CAD build for the part. Positions are in the model's coordinates, mm. A direction names the side the tool comes from. Give positions to 0.01 mm unless a question says otherwise; leave off trailing zeros. Order: outer loops, then holes, each group sorted by start corner. A loop starts at its lowest first (then second) coordinate and runs counter-clockwise, first axis right, second up. Notation, with made-up numbers: M 36,-17.5 L 67,-17.5 A25 ccw 67,-4.5 Z; hole C -19,35 d9. An arc over 180 degrees is marked long. Put each result on its own line as item: value. Start each with the question number.
1) Drill centre lines: line 1 (X direction, y = -157.7, z = 5.25); line 2 (X direction, y = -105, z = 0.75); line 3 (Y direction, x = 27, z = 8.25). Where is each one in solid material? Low to high. Write a range as [from, to].
2) Cut at A-A (x = 40). Write the cut outline in (y, z).
3) Cut at D-D (y = -104). Write the cut outline in (x, z).
4) Pin check, flat tips, straight feed: pin 1 (5 mm diameter, centred on x = -56.505, y = -54.325, fed in from -Z); pin 2 (1 mm diameter, centred on y = -138, z = 1, fed in from -X); pin 3 (1.5 mm diameter, centred on y = -124, z = 4, fed in from +X); pin 4 (5 mm diameter, centred on x = -52, z = 5, fed in from -Y). Stop position of each tip, or through.
5) Cut at C-C (z = 4.5). Give the number of separate pieces and of enclosed holes in the cut face, and give its area (3 significant figures).
6) Two-plate mould, pull along Y, no slides. Class faces 1 (the face through (-1, -23, 9.53)), 2 (the face through (62, -62.5, 5)), 3 (the face through (-38.85, -159.92, 4.83)): released by +Y, released by -Y, zero draft, split by the parting line, or undercut.
7) Cut at B-B (y = -157.7). Write the cut outline in (x, z), and give its area (3 significant figures).
8) Tool access for faces 4 (the face through (45, -115, 5)), 5 (the face through (-1, -23, 0)), 6 (the face through (-62, -62.5, 5)): list every direction of +Z, -Z, +X, -X, +Y, -Y with a clear straight run to the whole face (end or side of a thin tool).
```python
from build123d import *

# Parameters (mm, degrees)
RESSALTO_EXTRUS_O1_DEPTH = 9.53
CORTE_EXTRUS_O1_REACH    = 179.792
ESBO_O2_R                = 2.5
CORTE_EXTRUS_O2_REACH    = 179.792
ESBO_O3_R                = 1.5
CROQUIS1_W               = 1
CROQUIS1_H               = 125
SALIENTE_EXTRUIR1_DEPTH  = 9.53
REDONDEO1_R              = 6


with BuildPart() as part:
    # Esboço1 → Ressalto-extrusão1 (new body)
    with BuildSketch(Plane.XY):
        Polygon((-71.505, 62.5), (71.505, 62.5), (71.505, -62.5), (45, -62.5), (45, -162.5), (-45, -162.5), (-45, -62.5), (-71.505, -62.5), align=None)
    extrude(amount=RESSALTO_EXTRUS_O1_DEPTH)

    # Esboço2 → Corte-extrusão1 (cut, up to next)
    with BuildSketch(Plane.XY.offset(9.53), mode=Mode.PRIVATE) as corte_extrus_o1_sk1:
        with Locations((-40, -157.7)):
            Circle(ESBO_O2_R)
    corte_extrus_o1_tool1 = extrude(corte_extrus_o1_sk1.sketch, amount=-CORTE_EXTRUS_O1_REACH, mode=Mode.PRIVATE) & part.part
    # Esboço2 → Corte-extrusão1 (cut, up to next)
    with BuildSketch(Plane.XY.offset(9.53), mode=Mode.PRIVATE) as corte_extrus_o1_sk2:
        with Locations((-25, -157.7)):
            Circle(ESBO_O2_R)
    corte_extrus_o1_tool2 = extrude(corte_extrus_o1_sk2.sketch, amount=-CORTE_EXTRUS_O1_REACH, mode=Mode.PRIVATE) & part.part
    # Esboço2 → Corte-extrusão1 (cut, up to next)
    with BuildSketch(Plane.XY.offset(9.53), mode=Mode.PRIVATE) as corte_extrus_o1_sk3:
        with Locations((25, -157.7)):
            Circle(ESBO_O2_R)
    corte_extrus_o1_tool3 = extrude(corte_extrus_o1_sk3.sketch, amount=-CORTE_EXTRUS_O1_REACH, mode=Mode.PRIVATE) & part.part
    # Esboço2 → Corte-extrusão1 (cut, up to next)
    with BuildSketch(Plane.XY.offset(9.53), mode=Mode.PRIVATE) as corte_extrus_o1_sk4:
        with Locations((40, -157.7)):
            Circle(ESBO_O2_R)
    corte_extrus_o1_tool4 = extrude(corte_extrus_o1_sk4.sketch, amount=-CORTE_EXTRUS_O1_REACH, mode=Mode.PRIVATE) & part.part
    # Esboço2 → Corte-extrusão1 (cut, up to next)
    with BuildSketch(Plane.XY.offset(9.53), mode=Mode.PRIVATE) as corte_extrus_o1_sk5:
        with Locations((40, -98.2)):
            Circle(ESBO_O2_R)
    corte_extrus_o1_tool5 = extrude(corte_extrus_o1_sk5.sketch, amount=-CORTE_EXTRUS_O1_REACH, mode=Mode.PRIVATE) & part.part
    # Esboço2 → Corte-extrusão1 (cut, up to next)
    with BuildSketch(Plane.XY.offset(9.53), mode=Mode.PRIVATE) as corte_extrus_o1_sk6:
        with Locations((25, -98.2)):
            Circle(ESBO_O2_R)
    corte_extrus_o1_tool6 = extrude(corte_extrus_o1_sk6.sketch, amount=-CORTE_EXTRUS_O1_REACH, mode=Mode.PRIVATE) & part.part
    # Esboço2 → Corte-extrusão1 (cut, up to next)
    with BuildSketch(Plane.XY.offset(9.53), mode=Mode.PRIVATE) as corte_extrus_o1_sk7:
        with Locations((-25, -98.2)):
            Circle(ESBO_O2_R)
    corte_extrus_o1_tool7 = extrude(corte_extrus_o1_sk7.sketch, amount=-CORTE_EXTRUS_O1_REACH, mode=Mode.PRIVATE) & part.part
    # Esboço2 → Corte-extrusão1 (cut, up to next)
    with BuildSketch(Plane.XY.offset(9.53), mode=Mode.PRIVATE) as corte_extrus_o1_sk8:
        with Locations((-40, -98.2)):
            Circle(ESBO_O2_R)
    corte_extrus_o1_tool8 = extrude(corte_extrus_o1_sk8.sketch, amount=-CORTE_EXTRUS_O1_REACH, mode=Mode.PRIVATE) & part.part
    add(corte_extrus_o1_tool1.solids().sort_by_distance((-40, -157.7, 9.53))[0], mode=Mode.SUBTRACT)
    add(corte_extrus_o1_tool2.solids().sort_by_distance((-25, -157.7, 9.53))[0], mode=Mode.SUBTRACT)
    add(corte_extrus_o1_tool3.solids().sort_by_distance((25, -157.7, 9.53))[0], mode=Mode.SUBTRACT)
    add(corte_extrus_o1_tool4.solids().sort_by_distance((40, -157.7, 9.53))[0], mode=Mode.SUBTRACT)
    add(corte_extrus_o1_tool5.solids().sort_by_distance((40, -98.2, 9.53))[0], mode=Mode.SUBTRACT)
    add(corte_extrus_o1_tool6.solids().sort_by_distance((25, -98.2, 9.53))[0], mode=Mode.SUBTRACT)
    add(corte_extrus_o1_tool7.solids().sort_by_distance((-25, -98.2, 9.53))[0], mode=Mode.SUBTRACT)
    add(corte_extrus_o1_tool8.solids().sort_by_distance((-40, -98.2, 9.53))[0], mode=Mode.SUBTRACT)

    # Esboço3 → Corte-extrusão2 (cut, up to next)
    with BuildSketch(Plane(origin=(0, 0, 0), x_dir=(-1, 0, 0), z_dir=(0, 0, -1)), mode=Mode.PRIVATE) as corte_extrus_o2_sk1:
        with Locations((56.505, -54.325)):
            Circle(ESBO_O3_R)
    corte_extrus_o2_tool1 = extrude(corte_extrus_o2_sk1.sketch, amount=-CORTE_EXTRUS_O2_REACH, mode=Mode.PRIVATE) & part.part
    # Esboço3 → Corte-extrusão2 (cut, up to next)
    with BuildSketch(Plane(origin=(0, 0, 0), x_dir=(-1, 0, 0), z_dir=(0, 0, -1)), mode=Mode.PRIVATE) as corte_extrus_o2_sk2:
        with Locations((26.505, -54.325)):
            Circle(ESBO_O3_R)
    corte_extrus_o2_tool2 = extrude(corte_extrus_o2_sk2.sketch, amount=-CORTE_EXTRUS_O2_REACH, mode=Mode.PRIVATE) & part.part
    # Esboço3 → Corte-extrusão2 (cut, up to next)
    with BuildSketch(Plane(origin=(0, 0, 0), x_dir=(-1, 0, 0), z_dir=(0, 0, -1)), mode=Mode.PRIVATE) as corte_extrus_o2_sk3:
        with Locations((-26.505, -54.325)):
            Circle(ESBO_O3_R)
    corte_extrus_o2_tool3 = extrude(corte_extrus_o2_sk3.sketch, amount=-CORTE_EXTRUS_O2_REACH, mode=Mode.PRIVATE) & part.part
    # Esboço3 → Corte-extrusão2 (cut, up to next)
    with BuildSketch(Plane(origin=(0, 0, 0), x_dir=(-1, 0, 0), z_dir=(0, 0, -1)), mode=Mode.PRIVATE) as corte_extrus_o2_sk4:
        with Locations((-56.505, -54.325)):
            Circle(ESBO_O3_R)
    corte_extrus_o2_tool4 = extrude(corte_extrus_o2_sk4.sketch, amount=-CORTE_EXTRUS_O2_REACH, mode=Mode.PRIVATE) & part.part
    # Esboço3 → Corte-extrusão2 (cut, up to next)
    with BuildSketch(Plane(origin=(0, 0, 0), x_dir=(-1, 0, 0), z_dir=(0, 0, -1)), mode=Mode.PRIVATE) as corte_extrus_o2_sk5:
        with Locations((-56.423186497, 54.325)):
            Circle(ESBO_O3_R)
    corte_extrus_o2_tool5 = extrude(corte_extrus_o2_sk5.sketch, amount=-CORTE_EXTRUS_O2_REACH, mode=Mode.PRIVATE) & part.part
    # Esboço3 → Corte-extrusão2 (cut, up to next)
    with BuildSketch(Plane(origin=(0, 0, 0), x_dir=(-1, 0, 0), z_dir=(0, 0, -1)), mode=Mode.PRIVATE) as corte_extrus_o2_sk6:
        with Locations((-26.423186497, 54.325)):
            Circle(ESBO_O3_R)
    corte_extrus_o2_tool6 = extrude(corte_extrus_o2_sk6.sketch, amount=-CORTE_EXTRUS_O2_REACH, mode=Mode.PRIVATE) & part.part
    # Esboço3 → Corte-extrusão2 (cut, up to next)
    with BuildSketch(Plane(origin=(0, 0, 0), x_dir=(-1, 0, 0), z_dir=(0, 0, -1)), mode=Mode.PRIVATE) as corte_extrus_o2_sk7:
        with Locations((56.423186497, 54.325)):
            Circle(ESBO_O3_R)
    corte_extrus_o2_tool7 = extrude(corte_extrus_o2_sk7.sketch, amount=-CORTE_EXTRUS_O2_REACH, mode=Mode.PRIVATE) & part.part
    # Esboço3 → Corte-extrusão2 (cut, up to next)
    with BuildSketch(Plane(origin=(0, 0, 0), x_dir=(-1, 0, 0), z_dir=(0, 0, -1)), mode=Mode.PRIVATE) as corte_extrus_o2_sk8:
        with Locations((26.423186497, 54.325)):
            Circle(ESBO_O3_R)
    corte_extrus_o2_tool8 = extrude(corte_extrus_o2_sk8.sketch, amount=-CORTE_EXTRUS_O2_REACH, mode=Mode.PRIVATE) & part.part
    add(corte_extrus_o2_tool1.solids().sort_by_distance((-56.505, -54.325, 0))[0], mode=Mode.SUBTRACT)
    add(corte_extrus_o2_tool2.solids().sort_by_distance((-26.505, -54.325, 0))[0], mode=Mode.SUBTRACT)
    add(corte_extrus_o2_tool3.solids().sort_by_distance((26.505, -54.325, 0))[0], mode=Mode.SUBTRACT)
    add(corte_extrus_o2_tool4.solids().sort_by_distance((56.505, -54.325, 0))[0], mode=Mode.SUBTRACT)
    add(corte_extrus_o2_tool5.solids().sort_by_distance((56.423186, 54.325, 0))[0], mode=Mode.SUBTRACT)
    add(corte_extrus_o2_tool6.solids().sort_by_distance((26.423186, 54.325, 0))[0], mode=Mode.SUBTRACT)
    add(corte_extrus_o2_tool7.solids().sort_by_distance((-56.423186, 54.325, 0))[0], mode=Mode.SUBTRACT)
    add(corte_extrus_o2_tool8.solids().sort_by_distance((-26.423186, 54.325, 0))[0], mode=Mode.SUBTRACT)

    # Croquis1 → Saliente-Extruir1 (add)
    with BuildSketch(Plane.XY.offset(9.53)):
        with Locations((-72.005, 0)):
            Rectangle(CROQUIS1_W, CROQUIS1_H)
        with Locations((72.005, 0)):
            Rectangle(CROQUIS1_W, CROQUIS1_H)
    extrude(amount=-SALIENTE_EXTRUIR1_DEPTH)

    # Redondeo1
    redondeo1_edges = [part.edges().sort_by_distance(p)[0] for p in [
        (45, -62.5, 4.765),
        (-45, -62.5, 4.765),
    ]]
    fillet(redondeo1_edges, radius=REDONDEO1_R)


solid = part.part
```
Solution:
1. line 1: [-45, -42.5], [-37.5, -27.5], [-22.5, 22.5], [27.5, 37.5], [42.5, 45]
1. line 2: [-45, 45]
1. line 3: [-162.5, -159.2], [-156.2, -99.7], [-96.7, -55.74], [-52.91, 52.94], [55.71, 62.5]
2. outline: M -162.5,0 L -160.2,0 L -160.2,9.53 L -162.5,9.53 Z; M -155.2,0 L -100.7,0 L -100.7,9.53 L -155.2,9.53 Z; M -95.7,0 L 62.5,0 L 62.5,9.53 L -95.7,9.53 Z
3. outline: M -45,0 L 45,0 L 45,9.53 L -45,9.53 Z
4. pin 1: z = 0
4. pin 2: x = -45
4. pin 3: x = 45
4. pin 4: y = -62.69
5. separate pieces: 1
5. enclosed holes: 16
5. area: 26,900 mm²
6. face 1: zero draft
6. face 2: released by -Y
6. face 3: undercut
7. outline: M -45,0 L -42.5,0 L -42.5,9.53 L -45,9.53 Z; M -37.5,0 L -27.5,0 L -27.5,9.53 L -37.5,9.53 Z; M -22.5,0 L 22.5,0 L 22.5,9.53 L -22.5,9.53 Z; M 27.5,0 L 37.5,0 L 37.5,9.53 L 27.5,9.53 Z; M 42.5,0 L 45,0 L 45,9.53 L 42.5,9.53 Z
7. area: 667 mm²
8. face 4: +Z, -Z, +X, -Y
8. face 5: -Z, +X, -X, +Y, -Y
8. face 6: +Z, -Z, -X, -Y
